For this review, take the finished solid that the model builds, in its own axes (mm). A direction names the side the tool comes from. Give positions to 0.01 mm unless a question says otherwise; leave off trailing zeros. Order: outer loops, then holes, each group sorted by start corner. A loop starts at its lowest first (then second) coordinate and runs counter-clockwise, first axis right, second up. Notation, with made-up numbers: (67.25, 61) - (100.25, 61) arc R13 ccw to (100.25, 81) - close; hole circle Ø1 at (2.5, 78). An arc over 180 degrees is marked (long way). Use a Markdown table: item, result. Add a question column.
1) Wall thickness on L1, parallel to X at y = 7.8, z = 19.5; L2, parallel to X at y = 2.5, z = -14.5: over which ranges is each line inside the solid? List them lowest first.
2) We need section D-D on y = 4. Give the number of separate pieces and of enclosed holes in the cut face, then the cut area to 3 significant figures.
3) We need section C-C on x = 11. Write out the cut boundary in (y, z).
4) Clearance check with flat-ended pins moving along their axes: P1, Ø3, axis at x = 19.5, z = 19, coming from the -Y side; P2, Ø14, axis at x = 7.5, z = -5.5, coming from the +Y side; P3, Ø3.5, axis at y = 8, z = 19, coming from the +X side; P4, Ø2.5, axis at x = -19, y = 7, coming from the -Z side. State where each tip first meets the part, or that it passes through.
5) We need section A-A on z = -12.5. Write out the cut boundary in (x, y), then the cut area to 3 significant figures.
6) Mouldability with a two-part tool opening along X and no side actions: class faces 1 (the face through (16.65, 3, 20)), 2 (the face through (0, 3, 24.5)), 3 (the face through (-18.06, 3.45, -17.04)), 4 (the face through (-23.559, 2.958, 23.508)) as released by +X, released by -X, zero draft, split by the parting line, or undercut.
7) We need section B-B on x = 18.5. Write out the cut boundary in (y, z).
8) Machinability: for faces 5 (the face through (19, 5, -15.024)), 6 (the face through (22.35, 3, 19)), 7 (the face through (22.487, 7.479, -22.459)), 8 (the face through (-23, 7, 18)), which of the approach directions +Z, -Z, +X, -X, +Y, -Y give a long, thin tool a straight path to every point of the face, cutting with its end or side? Answer none if there is none.
```python
from build123d import *

# Parameters (mm, degrees)
EXTRUDE_1_DEPTH     = 6
SKETCH_1_3_R        = 1.75
EXTRUDE_1_2_DEPTH   = 9
CUT_EXTRUDE_1_DEPTH = 7
SKETCH_3_W          = 7.976009827
SKETCH_3_H          = 30.047980346
SKETCH_3_W_2        = 30.047980346
SKETCH_3_H_2        = 7.976009827
CUT_EXTRUDE_2_DEPTH = 8
CUT_EXTRUDE_3_DEPTH = 5


with BuildPart() as part:
    # 草图1 → Extrude 1 (new body)
    with BuildSketch(Plane(origin=(0, 0, 0), x_dir=(1, 0, 0), z_dir=(0, 1, 0))):
        with BuildLine():
            Line((-24.5, 21.2), (-24.5, -21.2))
            ThreePointArc((-24.5, -21.2), (-23.533452378, -23.533452378), (-21.2, -24.5))
            Line((-21.2, -24.5), (21.2, -24.5))
            ThreePointArc((21.2, -24.5), (23.533452378, -23.533452378), (24.5, -21.2))
            Line((24.5, -21.2), (24.5, 21.2))
            ThreePointArc((24.5, 21.2), (23.533452378, 23.533452378), (21.2, 24.5))
            Line((21.2, 24.5), (-21.2, 24.5))
            ThreePointArc((-21.2, 24.5), (-23.533452378, 23.533452378), (-24.5, 21.2))
        make_face()
        with BuildLine():
            Line((-23, 21.2), (-23, -21.2))
            ThreePointArc((-23, -21.2), (-22.472792206, -22.472792206), (-21.2, -23))
            Line((-21.2, -23), (21.2, -23))
            ThreePointArc((21.2, -23), (22.472792206, -22.472792206), (23, -21.2))
            Line((23, -21.2), (23, 21.2))
            ThreePointArc((23, 21.2), (22.472792206, 22.472792206), (21.2, 23))
            Line((21.2, 23), (-21.2, 23))
            ThreePointArc((-21.2, 23), (-22.472792206, 22.472792206), (-23, 21.2))
        make_face(mode=Mode.SUBTRACT)
    extrude(amount=EXTRUDE_1_DEPTH)

    # 草图1<3> → Extrude 1 2 (add)
    with BuildSketch(Plane(origin=(0, 0, 0), x_dir=(1, 0, 0), z_dir=(0, 1, 0))):
        with BuildLine():
            Line((-21.2, -23), (21.2, -23))
            ThreePointArc((21.2, -23), (22.472792206, -22.472792206), (23, -21.2))
            Line((23, -21.2), (23, 21.2))
            ThreePointArc((23, 21.2), (22.472792206, 22.472792206), (21.2, 23))
            Line((21.2, 23), (-21.2, 23))
            ThreePointArc((-21.2, 23), (-22.472792206, 22.472792206), (-23, 21.2))
            Line((-23, 21.2), (-23, -21.2))
            ThreePointArc((-23, -21.2), (-22.472792206, -22.472792206), (-21.2, -23))
        make_face()
        with Locations(Location((-19.5, 19.5, 0), (0, 0, 270))):
            Circle(SKETCH_1_3_R, mode=Mode.SUBTRACT)
        with Locations(Location((19.5, 19.5, 0), (0, 0, 270))):
            Circle(SKETCH_1_3_R, mode=Mode.SUBTRACT)
        with Locations(Location((19.5, -19.5, 0), (0, 0, 270))):
            Circle(SKETCH_1_3_R, mode=Mode.SUBTRACT)
        with Locations(Location((-19.5, -19.5, 0), (0, 0, 270))):
            Circle(SKETCH_1_3_R, mode=Mode.SUBTRACT)
    extrude(amount=EXTRUDE_1_2_DEPTH)

    # 草图2 → 切除-拉伸1 (cut)
    with BuildSketch(Plane.XZ):
        Polygon((22.35, 17.854551733), (22.35, 21.145448267), (19.5, 22.790896534), (16.65, 21.145448267), (16.65, 17.854551733), (19.5, 16.209103466), align=None)
        Polygon((-17.854551733, 22.35), (-21.145448267, 22.35), (-22.790896534, 19.5), (-21.145448267, 16.65), (-17.854551733, 16.65), (-16.209103466, 19.5), align=None)
        Polygon((17.854551733, -22.35), (21.145448267, -22.35), (22.790896534, -19.5), (21.145448267, -16.65), (17.854551733, -16.65), (16.209103466, -19.5), align=None)
        Polygon((-22.35, -17.854551733), (-22.35, -21.145448267), (-19.5, -22.790896534), (-16.65, -21.145448267), (-16.65, -17.854551733), (-19.5, -16.209103466), align=None)
    extrude(amount=-CUT_EXTRUDE_1_DEPTH, mode=Mode.SUBTRACT)

    # 草图3 → 切除-拉伸2 (cut)
    with BuildSketch(Plane(origin=(0, 9, 0), x_dir=(1, 0, 0), z_dir=(0, 1, 0))):
        with Locations((19.011995087, 0)):
            Rectangle(SKETCH_3_W, SKETCH_3_H)
        with Locations((0, 19.011995087)):
            Rectangle(SKETCH_3_W_2, SKETCH_3_H_2)
        Rectangle(SKETCH_3_W_2, SKETCH_3_H)
        with Locations((0, -19.011995087)):
            Rectangle(SKETCH_3_W_2, SKETCH_3_H_2)
        with Locations((-19.011995087, 0)):
            Rectangle(SKETCH_3_W, SKETCH_3_H)
    extrude(amount=-CUT_EXTRUDE_2_DEPTH, mode=Mode.SUBTRACT)

    # 草图5 → 切除-拉伸3 (cut)
    with BuildSketch(Plane(origin=(0, 0, 0), x_dir=(-1, 0, 0), z_dir=(0, -1, 0))):
        with BuildLine():
            Line((-6, -13.6), (-7, -13.6))
            ThreePointArc((-7, -13.6), (-7.707106781, -13.892893219), (-8, -14.6))
            Line((-8, -14.6), (-8, -15))
            ThreePointArc((-8, -15), (-7.707106781, -15.707106781), (-7, -16))
            Line((-7, -16), (-6, -16))
            ThreePointArc((-6, -16), (-5.292893219, -15.707106781), (-5, -15))
            Line((-5, -15), (-5, -14.6))
            ThreePointArc((-5, -14.6), (-5.292893219, -13.892893219), (-6, -13.6))
        make_face()
    extrude(amount=-CUT_EXTRUDE_3_DEPTH, mode=Mode.SUBTRACT)


solid = part.part
```
Checked values:
| question | item | result |
|---|---|---|
| 1 | L1 | -23 to -21.25, -17.75 to -15.02, 15.02 to 17.75, 21.25 to 23 |
| 1 | L2 | -24.5 to -23, 23 to 24.5 |
| 2 | separate pieces | 1 |
| 2 | enclosed holes | 5 |
| 2 | area | 418 mm² |
| 3 | outline | (0, -24.5) - (6, -24.5) - (6, -23) - (1, -23) - (1, 23) - (6, 23) - (6, 24.5) - (0, 24.5) - close |
| 4 | P1 | y = 7 |
| 4 | P2 | y = 1 |
| 4 | P3 | x = 23 |
| 4 | P4 | z = -24.5 |
| 5 | outline | (-24.5, 0) - (24.5, 0) - (24.5, 6) - (23, 6) - (23, 1) - (-23, 1) - (-23, 6) - (-24.5, 6) - close |
| 5 | area | 64.0 mm² |
| 6 | face 1 | undercut |
| 6 | face 2 | zero draft |
| 6 | face 3 | undercut |
| 6 | face 4 | released by -X |
| 7 | outline | (0, -24.5) - (6, -24.5) - (6, -23) - (9, -23) - (9, -20.94) - (7, -20.94) - (7, -22.35) - (0, -22.35) - close; (0, -16.65) - (7, -16.65) - (7, -18.06) - (9, -18.06) - (9, -15.02) - (1, -15.02) - (1, 15.02) - (9, 15.02) - (9, 18.06) - (7, 18.06) - (7, 16.79) - (0, 16.79) - close; (0, 22.21) - (7, 22.21) - (7, 20.94) - (9, 20.94) - (9, 23) - (6, 23) - (6, 24.5) - (0, 24.5) - close |
| 8 | face 5 | +Y |
| 8 | face 6 | -Y |
| 8 | face 7 | -Z, +X, +Y |
| 8 | face 8 | +Z, -Z, -X, +Y |
